from build123d import *

# Parameters (mm, degrees)
F1_DEPTH = 2
F6_DEPTH = 2


with BuildPart() as f1:
    # F0 (on Front) → F1 (new body)
    with BuildSketch(Plane.XZ):
        Polygon((5.1576569676, 2.7410463956), (0, 0), (5.1576569676, -2.7410463956), (10.3153139353, 0), align=None)
    extrude(amount=F1_DEPTH)


with BuildPart() as f6:
    # F5 (on face) → F6 (new body)
    with BuildSketch(Plane(origin=(-2.1093194974, -51.3742344161, 3.9689756511), x_dir=(-0.9991631758, 0.0407801704, -0.003150519), z_dir=(0.0409016879, 0.9961946981, -0.0769621688))):
        Polygon((0, 7.8918055439), (-4.3265928001, 0), (0, -7.8918055439), (4.3265928001, 0), align=None)
    extrude(amount=-F6_DEPTH)


solid = f6.part
Build history of the part. All positions in model axes, mm. Give positions to 0.01 mm unless a question says otherwise; leave off trailing zeros. Loops run counter-clockwise (first coordinate to the right, second up) from the corner with the lowest first, then second, coordinate; pieces in that order, holes last. Notation, with made-up numbers: (84.25, 88.25) -> (120.25, 88.25) arc R17 cw to (120.25, 105.25) -> close; hole circle Ø7 at (76, -4.5). An arc over 180 degrees is marked (long way). Answer in a Markdown table with one row per item.
Item 1: Flat gauge pin, fed straight in: P1, Ø1.5, axis at y = -52, z = 5, coming from the +X side. Where does the tip first touch, or does it go through?
Findings below:
| item | result |
|---|---|
| P1 | stops at x = 2.07 |
Item 2: Slice it at B-B on z = 5. Write the cut outline in (x, y).
Findings below:
| item | result |
|---|---|
| outline | (-6.03, -53.14) -> (1.66, -53.46) -> (1.65, -51.45) -> (-5.86, -51.14) -> close |
Item 3: Slice it at A-A on y = -51.7. Write the cut outline in (x, z).
Findings below:
| item | result |
|---|---|
| outline | (-6.45, 3.99) -> (-3.66, -1.07) -> (0.72, 1.25) -> (2.21, 3.99) -> (-2.15, 11.91) -> close |
Item 4: Slice it at C-C on x = -1.75. Write the cut outline in (y, z), plus the area to 3 significant figures.
Findings below:
| item | result |
|---|---|
| outline | (-53.93, -2.94) -> (-51.95, -3.24) -> (-50.83, 11.18) -> (-52.84, 11.19) -> close |
| area | 28.7 mm² |
Item 5: Probe line 1 along Z through (x, y) = (-2, -52.4); line 2 along Z through (x, y) = (-5, -52.7); line 3 along Y through (x, z) = (0.25, 6). List the from-to ranges inside material, lowest first. Write a range as [from, to].
Findings below:
| item | result |
|---|---|
| line 1 | z = [-3.63, 11.64] |
| line 2 | z = [1.36, 6.82] |
| line 3 | y = [-53.32, -51.31] |
